Check sheet for the drawn part. Datum: minimum x, y, z corner. Units: mm. A direction names the side the tool comes from. Coordinates: 2 decimals unless noted, no trailing zeros. Write each loop counter-clockwise with the first axis right and the second up, starting at its lowest first coordinate (ties: lowest second). Pieces come first, ordered by that corner, then holes. Notation, with made-up numbers: (64, -28.5) -> (79, -28.5) arc R35 cw to (79, 5.5) -> close; hole circle Ø6 at (-3.5, -35.75). An arc over 180 degrees is marked (long way). Answer in a Markdown table with one row per item. Add a question column.
Q1. Gauge pin test, flat ends, axial feed: P1, Ø6.5, axis at y = 18.5, z = 21, coming from the -X side (1 decimal); P2, Ø4, axis at x = 6.5, z = 24.5, coming from the +Y side (1 decimal); P3, Ø8, axis at y = 11, z = 25.5, coming from the -X side. Record the tip position at first contact, or that the pin passes through.
Q2. Thickness scan on line 1 (Y direction, x = 30.2, z = 10); line 2 (Y direction, x = 29.95, z = 50) (1 decimal); line 3 (Y direction, x = 3, z = 7) (1 decimal). Record the ranges inside material, lowest first.
Q3. Section check A-A, the plane z = 10. Count the separate pieces of the cut face and the enclosed holes in it.
Q4. Tool access check on the marked faces 1 and 2. Record the directions out of +Z, -Z, +X, -X, +Y, -Y that give a thin tool (end or side, any length) a straight path to the whole face; none if there is none.
Q5. Section check B-B, the plane x = 14. Record the boundary of the cut face in (y, z) (1 decimal).
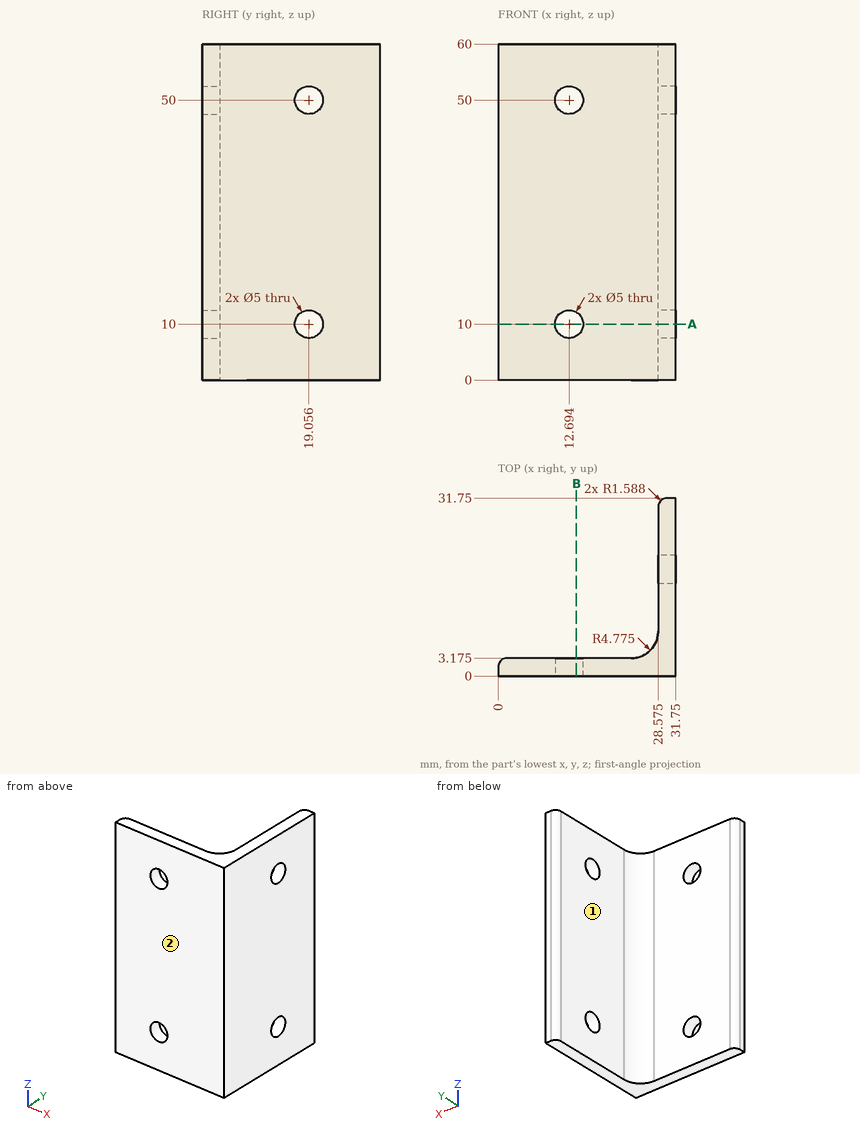
Calculated:
| question | item | result |
|---|---|---|
| 1 | P1 | stops at x = 28.6 |
| 1 | P2 | stops at y = 3.2 |
| 1 | P3 | stops at x = 28.48 |
| 2 | line 1 | y = 0 to 16.56, 21.56 to 31.75 |
| 2 | line 2 | y = 0 to 16.6, 21.6 to 31.7 |
| 2 | line 3 | y = 0 to 3.2 |
| 3 | separate pieces | 3 |
| 3 | enclosed holes | 0 |
| 4 | face 1 | +Z, -Z, -X, +Y |
| 4 | face 2 | +Z, -Z, +X, -X, -Y |
| 5 | outline | (0, 0) -> (3.2, 0) -> (3.2, 7.9) -> (0, 7.9) -> close; (0, 12.1) -> (3.2, 12.1) -> (3.2, 47.9) -> (0, 47.9) -> close; (0, 52.1) -> (3.2, 52.1) -> (3.2, 60) -> (0, 60) -> close |
